Verification items for the finished model (mm, model axes). A direction names the side the tool comes from. Coordinates: 2 decimals unless noted, no trailing zeros. Order: outer loops, then holes, each group sorted by start corner. A loop starts at its lowest first (then second) coordinate and runs counter-clockwise, first axis right, second up. Notation, with made-up numbers: M 25.25,84 L 82.25,84 A15 cw 82.25,108 Z; hole C 23.5,84 d6. An arc over 180 degrees is marked long. Return JSON: item names as keys, results as strings.
```python
from build123d import *

# Parameters (mm, degrees)
F1_DEPTH = 15
F2_W     = 1.381126
F2_H     = 2.695004
F3_DEPTH = 13.6


with BuildPart() as f1:
    # F0 (on Top) → F1 (new body)
    with BuildSketch(Plane.XY):
        with BuildLine():
            ThreePointArc((-7.5, 12.990381), (15, 0), (-7.5, -12.990381))
            Line((-7.5, -12.990381), (-10, -17.320508))
            ThreePointArc((-10, -17.320508), (5.352331, -19.27051), (17.5, -9.682458))
            Line((17.5, -9.682458), (22.5, -9.682458))
            Line((22.5, -9.682458), (22.5, 9.682458))
            Line((22.5, 9.682458), (17.5, 9.682458))
            ThreePointArc((17.5, 9.682458), (5.352331, 19.27051), (-10, 17.320508))
            Line((-10, 17.320508), (-7.5, 12.990381))
        make_face()
    extrude(amount=F1_DEPTH)

    # F2 (on face) → F3 (cut)
    with BuildSketch(Plane(origin=(0, 9.682458, 0), x_dir=(-1, 0, 0), z_dir=(0, 1, 0))):
        Polygon((-22.5, 6.152498), (-21.187555, 6.152498), (-21.187555, 3.439651), (-18.812445, 3.439651), (-18.812445, 11.560349), (-21.187555, 11.560349), (-21.187555, 8.847502), (-22.5, 8.847502), align=None)
        with Locations((-23.190563, 7.5)):
            Rectangle(F2_W, F2_H)
    extrude(amount=-F3_DEPTH, mode=Mode.SUBTRACT)


solid = f1.part
```
Q1. Cross-section at D-D, the plane y = -13.5. Record the boundary of the cut face in (x, z), and give its area (3 significant figures).
Values:
{"outline": "M -7.79,0 L -6.54,0 L -6.54,15 L -7.79,15 Z; M 6.54,0 L 14.76,0 L 14.76,15 L 6.54,15 Z", "area": "142 mm^2"}
Q2. Cross-section at C-C, the plane y = 0. Record the boundary of the cut face in (x, z).
Values:
{"outline": "M 15,0 L 22.5,0 L 22.5,6.15 L 21.19,6.15 L 21.19,3.44 L 18.81,3.44 L 18.81,11.56 L 21.19,11.56 L 21.19,8.85 L 22.5,8.85 L 22.5,15 L 15,15 Z"}
Q3. Material ranges on line 1 along Y through (x, z) = (0, 11.5); line 2 along X through (y, z) = (0, 10.25); line 3 along X through (y, z) = (0, 7.25), recorded low to high.
Values:
{"line 1": "-20 to -15, 15 to 20", "line 2": "15 to 18.81, 21.19 to 22.5", "line 3": "15 to 18.81"}
Q4. Go/stop test with flat-tipped pins: pin 1 (3 mm diameter, centred on y = 3.5, z = 10, fed in from -X); pin 2 (1.5 mm diameter, centred on x = 19, z = 6, fed in from +Y); pin 3 (3 mm diameter, centred on x = 12.5, z = 5.5, fed in from -Y). Record where each tip stops, or that it passes through.
Values:
{"pin 1": "x = 14.14", "pin 2": "y = 9.68", "pin 3": "y = -16.7"}
Q5. Tool access check on faces 4 (the face through (18, 9.682, 7)), 5 (the face through (20, 3, 11.56)), 6 (the face through (20, -9.682, 7)), 7 (the face through (22, 3, 8.848)), 8 (the face through (-8.77, 15.19, 7.4)). Record the directions out of +Z, -Z, +X, -X, +Y, -Y that give a thin tool (end or side, any length) a straight path to the whole face; none if there is none.
Values:
{"face 4": "+Z, -Z, +X, +Y", "face 5": "+Y", "face 6": "+Z, -Z, +X, -Y", "face 7": "+X, +Y", "face 8": "+Z, -Z, -X"}
Q6. Draft check along Z on faces 1 (the face through (15, 5, 0)), 2 (the face through (22, 3, 6.152)), 3 (the face through (-8.733, -15.125, 7.395)). Enter one of: pulls with the +Z half, pulls with the -Z half, needs draft (parallel to the pull), parting line crosses it, or undercut.
Values:
{"face 1": "pulls with the -Z half", "face 2": "undercut", "face 3": "needs draft"}
Q7. Cross-section at B-B, the plane z = 4.5. Record the boundary of the cut face in (x, y), and give its area (3 significant figures).
Values:
{"outline": "M -10,-17.32 A20 ccw 17.5,-9.68 L 22.5,-9.68 L 22.5,9.68 L 21.19,9.68 L 21.19,-3.92 L 18.81,-3.92 L 18.81,9.68 L 17.5,9.68 A20 ccw -10,17.32 L -7.5,12.99 A15 cw long -7.5,-12.99 Z", "area": "398 mm^2"}
Q8. Cross-section at A-A, the plane x = 0. Record the boundary of the cut face in (y, z), and give its area (3 significant figures).
Values:
{"outline": "M -20,0 L -15,0 L -15,15 L -20,15 Z; M 15,0 L 20,0 L 20,15 L 15,15 Z", "area": "150 mm^2"}
